Work out the finished part from the listing and answer in its coordinate system (mm). A direction names the side the tool comes from. Give positions to 0.01 mm unless a question says otherwise; leave off trailing zeros. Write each loop counter-clockwise with the first axis right and the second up, starting at its lowest first coordinate (ties: lowest second). Pieces come first, ordered by that corner, then holes. Notation, with made-up numbers: (67, 54) - (115, 54) arc R30 cw to (115, 80) - close; hole circle Ø6 at (-5, 85.25). An arc over 180 degrees is marked (long way). Write each question's results on one line, items separated by ' | '. Start each with the question number.
from build123d import *

# Parameters (mm, degrees)
F1_DEPTH = 381
F2_R     = 114.3
F3_DEPTH = 114.3
F4_R     = 114.3
F5_DEPTH = 157.48


with BuildPart() as f1:
    # F0 (on Front) → F1 (new body)
    with BuildSketch(Plane.XZ):
        with BuildLine():
            Line((-253.5002529621, -215.9), (0, -215.9))
            Line((0, -215.9), (0, -184.15))
            ThreePointArc((0, -184.15), (-158.75, -25.4), (0, 133.35))
            Line((0, 133.35), (0, 215.9))
            Line((0, 215.9), (-279.4, 54.6750131028))
            Line((-279.4, 54.6750131028), (-209.7759521092, -63.0383388986))
            ThreePointArc((-209.7759521092, -63.0383388986), (-204.5010974422, -75.4939283033), (-202.7002529621, -88.9))
            ThreePointArc((-202.7002529621, -88.9), (-217.5792284778, -124.8210244843), (-253.5002529621, -139.7))
            Line((-253.5002529621, -139.7), (-253.5002529621, -215.9))
        make_face()
        with BuildLine():
            Line((-279.4, -215.9), (-253.5002529621, -215.9))
            Line((-253.5002529621, -215.9), (-253.5002529621, -139.7))
            ThreePointArc((-253.5002529621, -139.7), (-266.9276691811, -137.8933107034), (-279.4, -132.6017517197))
            Line((-279.4, -132.6017517197), (-279.4, -215.9))
        make_face()
        with BuildLine():
            Line((0, -215.9), (279.4, -215.9))
            Line((279.4, -215.9), (279.4, -182.111337781))
            Line((279.4, -182.111337781), (279.4, -132.6017517197))
            ThreePointArc((279.4, -132.6017517197), (217.5948803765, -124.8366695659), (209.7759521092, -63.0383388986))
            Line((209.7759521092, -63.0383388986), (279.4, 54.6750131028))
            Line((279.4, 54.6750131028), (0, 215.9))
            Line((0, 215.9), (0, 133.35))
            ThreePointArc((0, 133.35), (112.2532015134, 86.8532015134), (158.75, -25.4))
            ThreePointArc((158.75, -25.4), (112.2532015134, -137.6532015134), (0, -184.15))
            Line((0, -184.15), (0, -215.9))
        make_face()
    extrude(amount=F1_DEPTH)

    # F2 (on face) → F3 (cut)
    with BuildSketch(Plane(origin=(93.4623118289, 0, 161.968503937), x_dir=(0.8661417323, 0, -0.499798459), z_dir=(0.499798459, 0, 0.8661417323))):
        with Locations((53.3835127066, -219.71)):
            Circle(F2_R)
    extrude(amount=-F3_DEPTH, mode=Mode.SUBTRACT)

    # F4 (on face) → F5 (cut)
    with BuildSketch(Plane(origin=(-93.4623118289, 0, 161.968503937), x_dir=(0.8661417323, 0, 0.499798459), z_dir=(-0.499798459, 0, 0.8661417323))):
        with Locations((-53.3835127066, -165.1)):
            Circle(F4_R)
    extrude(amount=-F5_DEPTH, mode=Mode.SUBTRACT)


solid = f1.part
Q1. A cutting plane is placed at B-B, the plane x = -76.5. Give the number of separate pieces and of enclosed holes in the cut face, and give its area (3 significant figures).
Q2. Given pin 1 (1 mm diameter, centred on y = -243.5, z = -104.5, fed in from +X); pin 2 (6 mm diameter, centred on x = 126.5, y = -146.5, fed in from +Z); pin 3 (5 mm diameter, centred on x = 89.5, y = -209.5, fed in from +Z), each flat-ended and moving along its own axis, determine where each tip first touches the part or whether it passes through.
Q3. A cutting plane is placed at A-A, the plane y = -24. Write down the section's boundary in (x, z), and give its area (3 significant figures).
Q4. Consider L1, parallel to Z at x = 0, y = -248; L2, parallel to X at y = -301.5, z = -25.4; L3, parallel to Y at x = -202.5, z = 92.5. Determine where each line is inside the solid, lowest interval first.
Q5. A cutting plane is placed at C-C, the plane y = -324. Write down the section's boundary in (x, z).
Q6. The mould has two halves that part along Z. Classify faces 4 (the flat face through (244.1, -187.83, -5.01)), 5 (the flat face through (-4, 0, -189)), 6 (the flat face through (-199.83, -272.5, 100.59)): pulls with the +Z half, pulls with the -Z half, needs draft (parallel to the pull), parting line crosses it, or undercut.
Q7. A tool of negligible diameter and unlimited length cuts with its end or side. For faces 1 (the flat face through (166.81, -218.67, -12.32)), 2 (the flat face through (-279.4, -188, -174)), 3 (the flat face through (-245.075, -187.833, -3.358)), from which of +Z, -Z, +X, -X, +Y, -Y can it reach the whole face along a straight path? Write none if from no direction.
Result:
1) separate pieces: 3 | enclosed holes: 0 | area: 30,400 mm2
2) pin 1: stops at x = 205.32 | pin 2: stops at z = -117.22 | pin 3: stops at z = -154.77
3) outline: (-279.4, -215.9) - (279.4, -215.9) - (279.4, -132.6) arc R50.8 cw to (209.78, -63.04) - (279.4, 54.68) - (0, 215.9) - (-279.4, 54.68) - (-209.78, -63.04) arc R50.8 cw to (-279.4, -132.6) - close; hole circle Ø317.5 at (0, -25.4) | area: 98,500 mm2
4) L1: z = -215.9 to -184.15, 133.35 to 215.9 | L2: x = -232.04 to -158.75, 158.75 to 232.04 | L3: y = -381 to -250.67, -79.53 to 0
5) outline: (-279.4, -215.9) - (279.4, -215.9) - (279.4, -132.6) arc R50.8 cw to (209.78, -63.04) - (279.4, 54.68) - (180.22, 111.91) - (141.97, 45.63) arc R158.75 cw (long way) to (74.01, 115.04) - (99.18, 158.67) - (0, 215.9) - (-279.4, 54.68) - (-209.78, -63.04) arc R50.8 cw to (-279.4, -132.6) - close
6) face 4: undercut | face 5: needs draft | face 6: pulls with the +Z half
7) face 1: +Z | face 2: +Z, -Z, -X, +Y, -Y | face 3: -X, +Y, -Y
